The model under review builds one solid part; all positions refer to its coordinate system, in mm. A direction names the side the tool comes from. Coordinates: 2 decimals unless noted, no trailing zeros. Loops run counter-clockwise (first coordinate to the right, second up) from the corner with the lowest first, then second, coordinate; pieces in that order, holes last. Notation, with made-up numbers: (-21, 87) - (23, 87) arc R13 cw to (23, 96) - close; hole circle Ø1 at (-18.5, 32). An arc over 180 degrees is marked (long way). Answer in a Markdown table with one row per item. Add a question column.
(1) For line 1 along X through (y, z) = (-15.75, 0); line 2 along Z through (x, y) = (2.25, -12.75), list the stretches that pass through material, from the lowest coordinate up.
(2) We need section A-A on y = -18. Write out the cut boundary in (x, z).
(3) We need section B-B on z = 0. Write out the cut boundary in (x, y).
(4) We need section C-C on y = -4.75. Write out the cut boundary in (x, z), plus the area to 3 significant figures.
(5) For P1, Ø6, axis at x = 1.5, z = -5, coming from the +Y side; P2, Ø2, axis at y = -17.5, z = 7.5, coming from the -X side; P3, Ø0.8, axis at y = -13.5, z = -7.5, coming from the -X side; P4, Ø8, axis at y = -18, z = 6, coming from the +X side, all flat-tipped, find the tip position at first contact; note any pin that passes through.
(6) Machinability: for faces 1 (the flat face through (-1.143, -16, 8)), 2 (the flat face through (5, 0, 5)), which of the approach directions +Z, -Z, +X, -X, +Y, -Y give a long, thin tool a straight path to every point of the face, cutting with its end or side? Answer none if there is none.
from build123d import *
from build123d import SkipClean  # not in build123d's __all__

# Parameters (mm, degrees)
F0_R     = 9.144
F0_R_2   = 6.604
F1_DEPTH = 10.922
F4_DEPTH = 9.652


with BuildPart() as f1:
    # F0 (on Front) → F1 (new body)
    with BuildSketch(Plane.XZ):
        Circle(F0_R)
        Circle(F0_R_2, mode=Mode.SUBTRACT)
    extrude(amount=F1_DEPTH)

    # F3 (on offset) → F4 (join)
    with BuildSketch(Plane.XZ.offset(20.574)):
        with BuildLine():
            Line((-1.143, 6.5043344779), (-1.143, 9.0722812456))
            ThreePointArc((-1.143, 9.0722812456), (-9.144, 0), (-1.143, -9.0722812456))
            Line((-1.143, -9.0722812456), (-1.143, -6.5043344779))
            ThreePointArc((-1.143, -6.5043344779), (-6.604, 0), (-1.143, 6.5043344779))
        make_face()
        with BuildLine():
            ThreePointArc((1.143, -9.0722812456), (9.144, 0), (1.143, 9.0722812456))
            Line((1.143, 9.0722812456), (1.143, 6.5043344779))
            ThreePointArc((1.143, 6.5043344779), (6.604, 0), (1.143, -6.5043344779))
            Line((1.143, -6.5043344779), (1.143, -9.0722812456))
        make_face()
    with SkipClean():  # cleaning this boolean's faces spoils the solid; the shape is the same uncleaned
        extrude(amount=-F4_DEPTH)


solid = f1.part
Outcome:
| question | item | result |
|---|---|---|
| 1 | line 1 | -9.14 to -6.6, 6.6 to 9.14 |
| 1 | line 2 | -8.86 to -6.21, 6.21 to 8.86 |
| 2 | outline | (-1.14, -9.07) - (-1.14, -6.5) arc R6.6 cw to (-1.14, 6.5) - (-1.14, 9.07) arc R9.14 ccw to start; (1.14, -9.07) arc R9.14 ccw to (1.14, 9.07) - (1.14, 6.5) arc R6.6 cw to (1.14, -6.5) - close |
| 3 | outline | (-9.14, -20.57) - (-6.6, -20.57) - (-6.6, 0) - (-9.14, 0) - close; (6.6, -20.57) - (9.14, -20.57) - (9.14, 0) - (6.6, 0) - close |
| 4 | outline | circle Ø18.29 at (0, 0); hole circle Ø13.21 at (0, 0) |
| 4 | area | 126 mm² |
| 5 | P1 | y = 0 |
| 5 | P2 | x = -6.43 |
| 5 | P3 | x = -5.76 |
| 5 | P4 | x = 8.92 |
| 6 | face 1 | +Z, -Z, -Y |
| 6 | face 2 | +Z, -Z, +X, -X, +Y |
